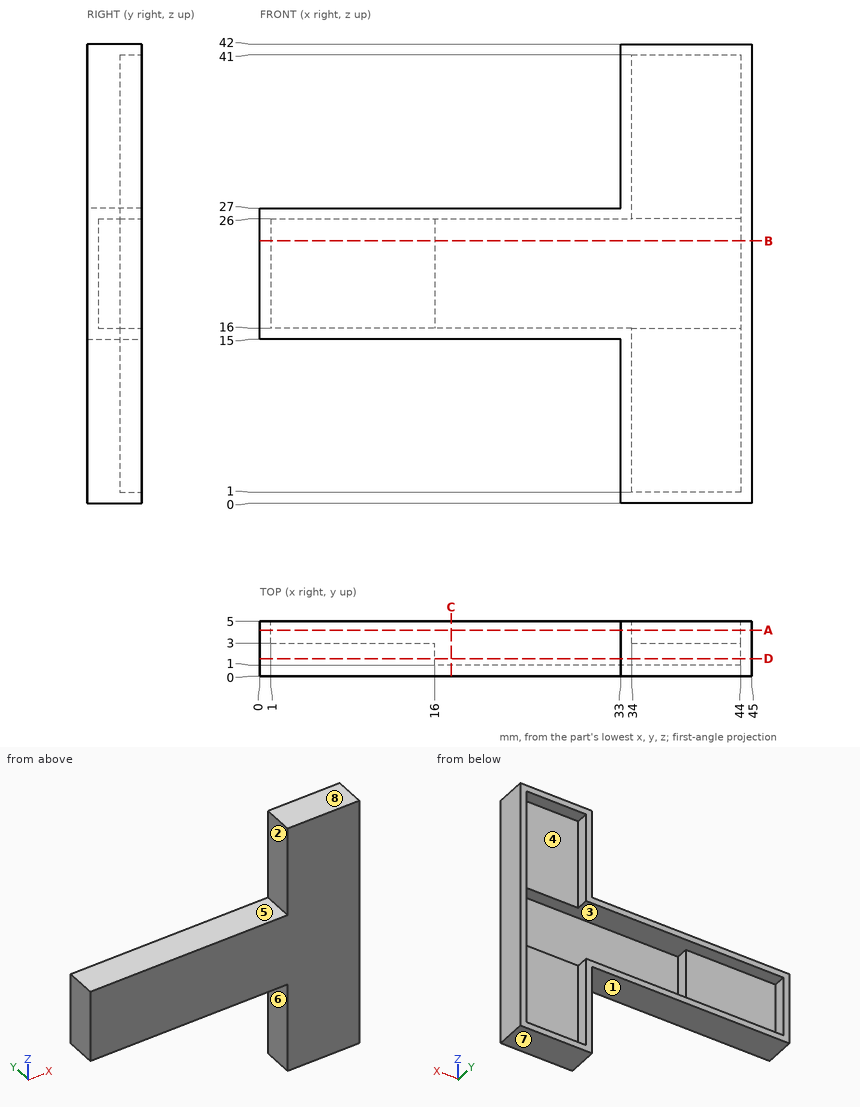
Print and shaded views of the part. All mm, measured from the part's lowest x, y and z. A direction names the side the tool comes from. Round coordinates to 2 decimals unless told otherwise and drop trailing zeros. Write each loop counter-clockwise with the first axis right and the second up, starting at its lowest first coordinate (ties: lowest second). Pieces come first, ordered by that corner, then holes. Notation, with made-up numbers: (11, 34) - (28, 34) arc R11 cw to (28, 40) - close; hole circle Ø1 at (-33, 52). An arc over 180 degrees is marked (long way). One line per question, with ' | ' between items.
1. Band-saw the part on B-B, the plane z = 24. Write the cut outline in (x, y).
Results are:
outline: (0, 0) - (45, 0) - (45, 5) - (44, 5) - (44, 1) - (16, 1) - (16, 3) - (1, 3) - (1, 5) - (0, 5) - close
2. Band-saw the part on A-A, the plane y = 4.2. Write the cut outline in (x, z), and give its area (3 significant figures).
Results are:
outline: (0, 15) - (33, 15) - (33, 0) - (45, 0) - (45, 42) - (33, 42) - (33, 27) - (0, 27) - close; hole (1, 16) - (34, 16) - (34, 1) - (44, 1) - (44, 41) - (34, 41) - (34, 26) - (1, 26) - close | area: 170 mm^2
3. Tool access for the marked faces 4, 5, 6, 7 and 8: list every direction of +Z, -Z, +X, -X, +Y, -Y with a clear straight run to the whole face (end or side of a thin tool).
Results are:
face 4: +Y | face 5: +Z, -X, +Y, -Y | face 6: -Z, -X, +Y, -Y | face 7: -Z, +X, -X, +Y, -Y | face 8: +Z, +X, -X, +Y, -Y
4. Band-saw the part on D-D, the plane y = 1.6. Write the cut outline in (x, z).
Results are:
outline: (0, 15) - (33, 15) - (33, 0) - (45, 0) - (45, 42) - (33, 42) - (33, 27) - (0, 27) - close; hole (16, 16) - (44, 16) - (44, 26) - (16, 26) - close
5. Band-saw the part on C-C, the plane x = 17.5. Write the cut outline in (y, z).
Results are:
outline: (0, 15) - (5, 15) - (5, 16) - (1, 16) - (1, 26) - (5, 26) - (5, 27) - (0, 27) - close
6. Drop flat-ended pins along their axis: pin 1 Ø1.2 at (y, z) = (3.5, 18) entering from -X; pin 2 Ø3 at (x, y) = (20, 3.5) entering from +Z; pin 3 Ø3 at (x, z) = (28.5, 22) entering from +Y; pin 4 Ø2 at (x, y) = (7.5, 4) entering from -Z. Give the stop position or say it passes through.
Results are:
pin 1: x = 0 | pin 2: z = 27 | pin 3: y = 1 | pin 4: z = 15
7. Mould opens along Z. For the marked faces 1, 2 and 3 say: released by +Z, released by -Z, zero draft, split by the parting line, or undercut.
Results are:
face 1: released by -Z | face 2: zero draft | face 3: undercut
8. Drill centre lines: line 1 along X through (y, z) = (2.2, 17); line 2 along X through (y, z) = (3.7, 3); line 3 along Z through (x, y) = (34, 2.6). Where is each one in solid material? Low to high. Write a range as from..to.
Results are:
line 1: 0..16, 44..45 | line 2: 33..34, 44..45 | line 3: 0..16, 26..42
